Work out the finished part from the listing and answer in its coordinate system (mm). Face numbers are marked on the shaded views. A direction names the side the tool comes from. Coordinates: 2 decimals unless noted, no trailing zeros. Order: outer loops, then holes, each group sorted by start corner. A loop starts at its lowest first (then second) coordinate and runs counter-clockwise, first axis right, second up. Notation, with made-up numbers: M 71,0 L 92,0 A23 ccw 92,21 Z; hole C 31.5,-37 d11. An arc over 180 degrees is marked long. Use a Markdown table: item, result.
from build123d import *

# Parameters (mm, degrees)
SKETCH_1_R      = 12
SKETCH_1_R_2    = 10
SKETCH_1_R_3    = 7
EXTRUDE_1_DEPTH = 311


with BuildPart() as part:
    # Эскиз1 → Бобышка-Вытянуть1 (new body)
    with BuildSketch(Plane.XY):
        with BuildLine():
            ThreePointArc((-37.98749513, -35.509860796), (17.746819787, -48.877913084), (51.920988797, -2.865470704))
            Line((51.920988797, -2.865470704), (61.180982268, 109.607242119))
            ThreePointArc((61.180982268, 109.607242119), (38.277381578, 148.980209754), (-6.912328256, 143.262200477))
            ThreePointArc((-6.912328256, 143.262200477), (-15.936398986, 137.913716983), (-26.250179642, 135.999022019))
            ThreePointArc((-26.250179642, 135.999022019), (-41.620493207, 131.928483524), (-53.134256146, 120.962669112))
            ThreePointArc((-53.134256146, 120.962669112), (-72.149102751, 40.15262637), (-37.98749513, -35.509860796))
        make_face()
        with BuildLine():
            ThreePointArc((-11.523694148, -7.950124099), (-8.228993532, -11.326237921), (-4, -13.416407865))
            Line((-4, -13.416407865), (-4, -21.583592135))
            ThreePointArc((-4, -21.583592135), (-10.327212311, -25.547556618), (-13.71714256, -32.2))
            ThreePointArc((-13.71714256, -32.2), (-20.57248383, -28.315594803), (-26.38518966, -22.996125035))
            ThreePointArc((-26.38518966, -22.996125035), (-21.105886088, -17.716391723), (-19.291147968, -10.473922835))
            Line((-19.291147968, -10.473922835), (-11.523694148, -7.950124099))
        make_face(mode=Mode.SUBTRACT)
        with Locations((-56, 34)):
            Circle(SKETCH_1_R, mode=Mode.SUBTRACT)
        with BuildLine():
            ThreePointArc((-11.122034659, 8.502960957), (-13.314791228, 4.326237921), (-13.995830103, -0.341671969))
            Line((-13.995830103, -0.341671969), (-21.763283923, -2.865470704))
            ThreePointArc((-21.763283923, -2.865470704), (-27.488454305, 1.927133403), (-34.86284999, 3.095430597))
            ThreePointArc((-34.86284999, 3.095430597), (-33.28697807, 10.815594803), (-30.024086569, 17.987613119))
            ThreePointArc((-30.024086569, 17.987613119), (-23.371367276, 14.598224375), (-15.922585126, 15.110351828))
            Line((-15.922585126, 15.110351828), (-11.122034659, 8.502960957))
        make_face(mode=Mode.SUBTRACT)
        with BuildLine():
            Line((4, -21.583592135), (4, -13.416407865))
            ThreePointArc((4, -13.416407865), (8.228993532, -11.326237921), (11.523694148, -7.950124099))
            Line((11.523694148, -7.950124099), (19.291147968, -10.473922835))
            ThreePointArc((19.291147968, -10.473922835), (21.105886088, -17.716391723), (26.38518966, -22.996125035))
            ThreePointArc((26.38518966, -22.996125035), (20.57248383, -28.315594803), (13.71714256, -32.2))
            ThreePointArc((13.71714256, -32.2), (10.327212311, -25.547556618), (4, -21.583592135))
        make_face(mode=Mode.SUBTRACT)
        with BuildLine():
            ThreePointArc((4.649898704, 13.205242975), (0, 14), (-4.649898704, 13.205242975))
            Line((-4.649898704, 13.205242975), (-9.450449171, 19.812633846))
            ThreePointArc((-9.450449171, 19.812633846), (-6.661586748, 26.738590562), (-7.829283679, 34.113081319))
            ThreePointArc((-7.829283679, 34.113081319), (0, 35), (7.829283679, 34.113081319))
            ThreePointArc((7.829283679, 34.113081319), (6.661586748, 26.738590562), (9.450449171, 19.812633846))
            Line((9.450449171, 19.812633846), (4.649898704, 13.205242975))
        make_face(mode=Mode.SUBTRACT)
        with BuildLine():
            ThreePointArc((13.995830103, -0.341671969), (13.314791228, 4.326237921), (11.122034659, 8.502960957))
            Line((11.122034659, 8.502960957), (15.922585126, 15.110351828))
            ThreePointArc((15.922585126, 15.110351828), (23.371367276, 14.598224375), (30.024086569, 17.987613119))
            ThreePointArc((30.024086569, 17.987613119), (33.28697807, 10.815594803), (34.86284999, 3.095430597))
            ThreePointArc((34.86284999, 3.095430597), (27.488454305, 1.927133403), (21.763283923, -2.865470704))
            Line((21.763283923, -2.865470704), (13.995830103, -0.341671969))
        make_face(mode=Mode.SUBTRACT)
        with Locations((38, 44)):
            Circle(SKETCH_1_R_2, mode=Mode.SUBTRACT)
        with Locations((-26, 85)):
            Circle(SKETCH_1_R_3, mode=Mode.SUBTRACT)
        with BuildLine():
            ThreePointArc((-39.719957497, 75.210764299), (-29.341451826, 72.9489184), (-18.758284903, 73.857711393))
            ThreePointArc((-18.758284903, 73.857711393), (1.170574134, 89.074856744), (3.323461498, 114.056570279))
            ThreePointArc((3.323461498, 114.056570279), (6.219388218, 129.16434937), (20, 136))
            ThreePointArc((20, 136), (39.428131569, 126.090695644), (42.812990739, 104.545641977))
            ThreePointArc((42.812990739, 104.545641977), (8.162699165, 61.508737426), (-46.303776516, 52.223217173))
            ThreePointArc((-46.303776516, 52.223217173), (-55.536170835, 67.30405243), (-39.719957497, 75.210764299))
        make_face(mode=Mode.SUBTRACT)
        with Locations((-42.454482672, 113.5)):
            Circle(SKETCH_1_R_3, mode=Mode.SUBTRACT)
        with Locations((-26, 104)):
            Circle(SKETCH_1_R_3, mode=Mode.SUBTRACT)
        with Locations((-9.545517328, 113.5)):
            Circle(SKETCH_1_R_3, mode=Mode.SUBTRACT)
    extrude(amount=EXTRUDE_1_DEPTH)


solid = part.part
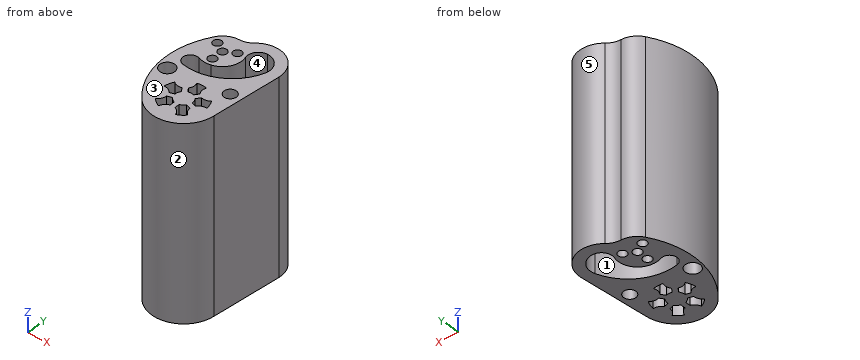
(1) Which of the six approach directions +Z, -Z, +X, -X, +Y, -Y give full straight-line access (tool end or side, diameter ignored) to the marked faces 1 and 2?
Conclusion:
| item | result |
|---|---|
| face 1 | +Z, -Z |
| face 2 | +Z, -Z, -Y |
(2) A cutting plane is placed at B-B (x = -62). Determine the outline of the cut face in (y, z).
Conclusion:
| item | result |
|---|---|
| outline | M 1.03,0 L 23.61,0 L 23.61,311 L 1.03,311 Z; M 44.39,0 L 104.14,0 L 104.14,311 L 44.39,311 Z |
(3) A cutting plane is placed at D-D (z = 265.5). Give the number of separate pieces and of enclosed holes in the cut face, then the cut area to 3 significant figures.
Conclusion:
| item | result |
|---|---|
| separate pieces | 1 |
| enclosed holes | 12 |
| area | 15,300 mm2 |
(4) Straight lines are drawn through the part: L1, parallel to X at y = 113, z = 235; L2, parallel to Y at x = 15.5, z = 295; L3, parallel to Y at x = -38.5, z = 61.5. For each, find the intervals that lie inside material, in ascending order.
Conclusion:
| item | result |
|---|---|
| L1 | -57.73 to -49.44, -35.47 to -16.53, -2.56 to 3.66, 43.98 to 61.24 |
| L2 | -49.64 to -31.38, -9.24 to -0.83, 14.53 to 66.39, 135.4 to 153 |
| L3 | -34.96 to 51.1, 74.77 to 107.72, 119.28 to 133.46 |
(5) A cutting plane is placed at C-C (y = 130). Determine the outline of the cut face in (x, z), then the cut area to 3 significant figures.
Conclusion:
| item | result |
|---|---|
| outline | M -44.65,0 L 6.9,0 L 6.9,311 L -44.65,311 Z; M 35.87,0 L 57.12,0 L 57.12,311 L 35.87,311 Z |
| area | 22,600 mm2 |
(6) Given P1, Ø8, axis at x = 22.5, z = 59, coming from the -Y side; P2, Ø6, axis at x = -37, z = 243.5, coming from the -Y side; P3, Ø8, axis at y = 80.5, z = 191.5, coming from the -X side, each flat-ended and moving along its own axis, determine where each tip first touches the part or whether it passes through.
Conclusion:
| item | result |
|---|---|
| P1 | y = -48.6 |
| P2 | y = -39.34 |
| P3 | x = -70.51 |
(7) Determine the mould class of the marked faces 3, 4 and 5 for opening direction X: pulls with the +X half, pulls with the -X half, needs draft (parallel to the pull), parting line crosses it, or undercut.
Conclusion:
| item | result |
|---|---|
| face 3 | needs draft |
| face 4 | undercut |
| face 5 | parting line crosses it |
(8) A cutting plane is placed at A-A (y = 85). Determine the outline of the cut face in (x, z).
Conclusion:
| item | result |
|---|---|
| outline | M -68.61,0 L -33,0 L -33,311 L -68.61,311 Z; M -19,0 L -1.51,0 L -1.51,311 L -19,311 Z; M 33.23,0 L 59.16,0 L 59.16,311 L 33.23,311 Z |
